The model under review builds one solid part; all positions refer to its coordinate system, in mm. A direction names the side the tool comes from. Round coordinates to 2 decimals unless told otherwise and drop trailing zeros. Order: outer loops, then holes, each group sorted by start corner. A loop starts at its lowest first (then second) coordinate and runs counter-clockwise, first axis right, second up. Notation, with made-up numbers: M -26,42.25 L -17,42.25 A32 ccw -17,78.25 Z; hole C -15.5,50 d1. An arc over 180 degrees is marked long. Answer as CSV lines item,"result". Start each with the question number.
from build123d import *

# Parameters (mm, degrees)
SKETCH_1_W                      = 28
SKETCH_1_H                      = 28
SKETCH_1_W_2                    = 19.9
SKETCH_1_H_2                    = 19.9
EXTRUDE_1_DEPTH                 = 20
CUT_EXTRUDE_1_DEPTH             = 20
SKETCH_3_W                      = 20
SKETCH_3_H                      = 4.05
EXTRUDE_2_DEPTH                 = 20
CUT_EXTRUDE_2_REACH             = 48.148
SKETCH_4_R                      = 1.8
CUT_EXTRUDE_2_DIRECTION_2_REACH = 48.148
SKETCH_5_W                      = 60
SKETCH_5_H                      = 100
EXTRUDE_3_DEPTH                 = 10
SKETCH_6_W                      = 10
SKETCH_6_H                      = 10
EXTRUDE_4_DEPTH                 = 60
CUT_EXTRUDE_3_REACH             = 96.345
SKETCH_8_W                      = 50
SKETCH_8_H                      = 90
CUT_EXTRUDE_4_DEPTH             = 1


with BuildPart() as part:
    # 草图1 → 凸台-拉伸1 (new body)
    with BuildSketch(Plane(origin=(0, 0, 0), x_dir=(1, 0, 0), z_dir=(0, 1, 0))):
        Rectangle(SKETCH_1_W, SKETCH_1_H)
        Rectangle(SKETCH_1_W_2, SKETCH_1_H_2, mode=Mode.SUBTRACT)
    extrude(amount=EXTRUDE_1_DEPTH)

    # 草图2 → 切除-拉伸1 (cut)
    with BuildSketch(Plane(origin=(0, 20, 0), x_dir=(1, 0, 0), z_dir=(0, 1, 0))):
        Polygon((14, 9.95), (9.95, 7.95), (9.95, -7.95), (14, -9.95), align=None)
    extrude(amount=-CUT_EXTRUDE_1_DEPTH, mode=Mode.SUBTRACT)

    # 草图3 → 凸台-拉伸2 (add)
    with BuildSketch(Plane(origin=(0, 20, 0), x_dir=(1, 0, 0), z_dir=(0, 1, 0))):
        with Locations((24, 11.975)):
            Rectangle(SKETCH_3_W, SKETCH_3_H)
        with Locations((24, -11.975)):
            Rectangle(SKETCH_3_W, SKETCH_3_H)
    extrude(amount=-EXTRUDE_2_DEPTH)

    # 草图4 → 切除-拉伸2 (cut, up to next)
    with BuildSketch(Plane.XY.offset(-9.95), mode=Mode.PRIVATE) as cut_extrude_2_sk1:
        with Locations((25, 10)):
            Circle(SKETCH_4_R)
    cut_extrude_2_tool1 = extrude(cut_extrude_2_sk1.sketch, amount=-CUT_EXTRUDE_2_REACH, mode=Mode.PRIVATE) & part.part
    add(cut_extrude_2_tool1.solids().sort_by_distance((25, 10, -9.95))[0], mode=Mode.SUBTRACT)

    # 切除-拉伸2 direction 2: up to this face of the body (flat: up to its plane)
    cut_extrude_2_direction_2_end = Plane(part.part.faces().sort_by_distance((10, 10, 14))[0])
    # 草图4 → 切除-拉伸2 direction 2 (cut, up to the picked face)
    with BuildSketch(Plane.XY.offset(-9.95), mode=Mode.PRIVATE) as cut_extrude_2_direction_2_sk1:
        with Locations((25, 10)):
            Circle(SKETCH_4_R)
    cut_extrude_2_direction_2_tool1 = split(extrude(cut_extrude_2_direction_2_sk1.sketch, amount=CUT_EXTRUDE_2_DIRECTION_2_REACH, mode=Mode.PRIVATE), bisect_by=cut_extrude_2_direction_2_end, keep=Keep.BOTH, mode=Mode.PRIVATE)
    add(cut_extrude_2_direction_2_tool1.solids().sort_by(Axis((25, 10, -9.95), (0, 0, 1)))[0], mode=Mode.SUBTRACT)

    # 草图5 → 凸台-拉伸3 (add)
    with BuildSketch(Plane(origin=(0, 20, 0), x_dir=(1, 0, 0), z_dir=(0, 1, 0))):
        with Locations((-44, 0)):
            Rectangle(SKETCH_5_W, SKETCH_5_H)
    extrude(amount=-EXTRUDE_3_DEPTH)

    # 草图6 → 凸台-拉伸4 (add)
    with BuildSketch(Plane.ZY.offset(14)):
        with Locations((0, 5)):
            Rectangle(SKETCH_6_W, SKETCH_6_H)
    extrude(amount=EXTRUDE_4_DEPTH)

    # 草图7 → 切除-拉伸3 (cut, up to next)
    with BuildSketch(Plane.XY.offset(5), mode=Mode.PRIVATE) as cut_extrude_3_sk1:
        Polygon((-74, 10), (-74, 0), (-14, 0), align=None)
    cut_extrude_3_tool1 = extrude(cut_extrude_3_sk1.sketch, amount=-CUT_EXTRUDE_3_REACH, mode=Mode.PRIVATE) & part.part
    add(cut_extrude_3_tool1.solids().sort_by_distance((-54, 3.333333, 5))[0], mode=Mode.SUBTRACT)

    # 草图8 → 切除-拉伸4 (cut)
    with BuildSketch(Plane(origin=(0, 20, 0), x_dir=(1, 0, 0), z_dir=(0, 1, 0))):
        with Locations((-44, 0)):
            Rectangle(SKETCH_8_W, SKETCH_8_H)
    extrude(amount=-CUT_EXTRUDE_4_DEPTH, mode=Mode.SUBTRACT)


solid = part.part
Item 1: Consider section C-C (y = 4). State the section outline as (x, z) points, and give its area (3 significant figures).
Item 2: The part is to be moulded in two halves that separate along Z. For faces 5 (the flat face through (-9.95, 10, 0)), 6 (the flat face through (-44, 5, 0)), 7 (the flat face through (10, 10, 14)), say which applies: +Z half, -Z half, draft (parallel to the pull), parting line (faces both ways), or undercut.
Item 3: Tool access review of faces 1 (the flat face through (-44, 10, -28)), 2 (the flat face through (10, 10, -14)), 3 (the flat face through (-14, 5, 10)), 4 (the flat face through (22, 10, 9.95)): name each direction out of +Z, -Z, +X, -X, +Y, -Y from which nothing blocks a thin tool from reaching the whole face with its end or side.
Item 4: Consider section D-D (x = 25). State the section outline as (y, z) points.
Item 5: For pin 1 (2 mm diameter, centred on x = 25, y = 10, fed in from +Z); pin 2 (1.5 mm diameter, centred on x = -19.5, z = -13.5, fed in from -Y); pin 3 (2 mm diameter, centred on y = 5.5, z = -9, fed in from -X); pin 4 (3 mm diameter, centred on x = -49.5, y = 7.5, fed in from +Z), all flat-tipped, find the tip position at first contact; note any pin that passes through.
Item 6: Consider section A-A (x = -2). State the section outline as (y, z) points, and give its area (3 significant figures).
Item 7: Consider section B-B (z = -12.5). State the section outline as (x, y) points, and give its area (3 significant figures).
Item 8: Wall thickness on probe 1 along Z at (x, y) = (-5, 5.5); probe 2 along Y at (x, z) = (25, 10.9); probe 3 along Z at (x, y) = (-50, 19.25): over which ranges is each line inside the solid? List them lowest first. Write a range as [from, to].
Reported:
1,outline,"M -38,-5 L -14,-5 L -14,-14 L 34,-14 L 34,-9.95 L 14,-9.95 L 9.95,-7.95 L 9.95,-9.95 L -9.95,-9.95 L -9.95,9.95 L 9.95,9.95 L 9.95,7.95 L 14,9.95 L 34,9.95 L 34,14 L -14,14 L -14,5 L -38,5 Z"
1,area,"717 mm²"
2,face 5,"undercut"
2,face 6,"draft"
2,face 7,"+Z half"
3,face 1,"-Z, -X, -Y"
3,face 2,"-Z, +X, +Y, -Y"
3,face 3,"+Z, -X, -Y"
3,face 4,"+X, +Y, -Y"
4,outline,"M 0,-14 L 8.2,-14 L 8.2,-9.95 L 0,-9.95 Z; M 0,9.95 L 8.2,9.95 L 8.2,14 L 0,14 Z; M 11.8,-14 L 20,-14 L 20,-9.95 L 11.8,-9.95 Z; M 11.8,9.95 L 20,9.95 L 20,14 L 11.8,14 Z"
5,pin 1,"passes through"
5,pin 2,"stops at y = 10"
5,pin 3,"stops at x = -14"
5,pin 4,"stops at z = 5"
6,outline,"M 0,-14 L 20,-14 L 20,-9.95 L 0,-9.95 Z; M 0,9.95 L 20,9.95 L 20,14 L 0,14 Z"
6,area,"162 mm²"
7,outline,"M -74,10 L -14,10 L -14,0 L 34,0 L 34,20 L -19,20 L -19,19 L -69,19 L -69,20 L -74,20 Z; hole C 25,10 d3.6"
7,area,"1,500 mm²"
8,probe 1,"z = [-14, -9.95], [9.95, 14]"
8,probe 2,"y = [0, 8.2], [11.8, 20]"
8,probe 3,"z = [-50, -45], [45, 50]"
